```python
from build123d import *

# Parameters (mm, degrees)
F3_R = 5


# Not quite as in the source:
# - a fillet or chamfer that OpenCascade refuses, or shapes differently, is made with other operations: its cross-section is extruded or revolved along the edge and cut away or added


with BuildPart() as f1:
    # F0 (on Front) → F1 (revolve)
    with BuildSketch(Plane.XZ):
        Polygon((4, 11.2420413941), (2, 11.2420413941), (1.5147400554, 6.2420413941), (2, 1.2420413941), (4, 1.2420413941), (2.3485091515, 6.2420413941), align=None)
    revolve(axis=Axis((0, 0, 6.2420413941), (0, 0, 1)))

    # F2: fillet of radius 1.5 on 2 edges, made by hand

    # F2_s1 → F2_t2 (revolve, cut)
    with BuildSketch(Plane.XZ):
        with BuildLine():
            ThreePointArc((3.3497763701, 9.2734454721), (3.162587688, 10.592136722), (2, 11.2420413941))
            Line((2, 11.2420413941), (4, 11.2420413941))
            Line((4, 11.2420413941), (3.3497763701, 9.2734454721))
        make_face()
    revolve(axis=Axis((0, 0, 11.2420413941), (0, 0, 1)), mode=Mode.SUBTRACT)

    # F2_s3 → F2_t4 (revolve, cut)
    with BuildSketch(Plane.XZ):
        with BuildLine():
            ThreePointArc((2, 1.2420413941), (3.162587688, 1.8919460662), (3.3497763701, 3.2106373161))
            Line((3.3497763701, 3.2106373161), (4, 1.2420413941))
            Line((4, 1.2420413941), (2, 1.2420413941))
        make_face()
    revolve(axis=Axis((0, 0, 1.2420413941), (0, 0, 1)), mode=Mode.SUBTRACT)

    # F3
    f3_edges = [f1.edges().sort_by_distance(p)[0] for p in [
        (-2.348509, 0, 6.242041),
    ]]
    fillet(f3_edges, radius=F3_R)


solid = f1.part
```
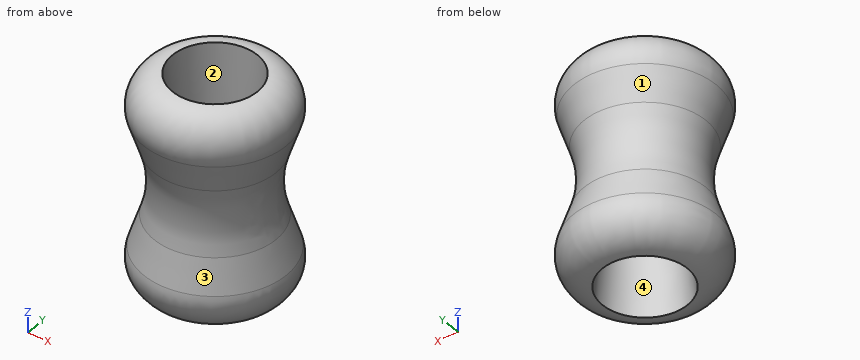
Geometry check sheet. Reference: the model listing, model coordinates, mm. Face numbers are marked on the shaded views. A direction names the side the tool comes from. Coordinates: 2 decimals unless noted, no trailing zeros. Order: outer loops, then holes, each group sorted by start corner. A loop starts at its lowest first (then second) coordinate and runs counter-clockwise, first axis right, second up. Notation, with made-up numbers: M -23,88 L 16,88 A28 ccw 16,106 Z; hole C -28,-28.75 d10. An arc over 180 degrees is marked long. Answer as a JSON object with one key per item and string values.
Q1. Cross-section at A-A on z = 8.25. Record the cut outline in (x, y), and give its area (3 significant figures).
Results are:
{"outline": "C 0,0 d6.02; hole C 0,0 d3.42", "area": "19.3 mm²"}
Q2. Tool access check on the marked faces 1 and 2. Record the directions out of +Z, -Z, +X, -X, +Y, -Y that give a thin tool (end or side, any length) a straight path to the whole face; none if there is none.
Results are:
{"face 1": "none", "face 2": "+Z"}
Q3. Cross-section at B-B on z = 3.75. Record the cut outline in (x, y).
Results are:
{"outline": "C 0,0 d6.34; hole C 0,0 d3.51"}
Q4. Scan lines: line 1 (X direction, y = -0.5, z = 2.25); line 2 (Y direction, x = -0.75, z = 5.25); line 3 (Y direction, x = -1.25, z = 8.75). Record each from-to range of solid material in increasing order.
Results are:
{"line 1": "x = -3.31 to -1.84, 1.84 to 3.31", "line 2": "y = -2.61 to -1.43, 1.43 to 2.61", "line 3": "y = -2.92 to -1.24, 1.24 to 2.92"}
Q5. Depth check by flat-ended pin: pin 1 Ø3 at (y, z) = (-1.5, 7) entering from -X; pin 2 Ø2 at (x, z) = (-2.5, 7) entering from -Y; pin 3 Ø1.5 at (y, z) = (0.5, 8) entering from +X. Enter the tip coordinate at first touch or a pass-through.
Results are:
{"pin 1": "stops at x = -2.94", "pin 2": "stops at y = -2.25", "pin 3": "stops at x = 3.15"}
Q6. Release check for a two-part mould opening along X. For the marked faces 3 and 4 record: released by +X, released by -X, zero draft, split by the parting line, or undercut.
Results are:
{"face 3": "split by the parting line", "face 4": "undercut"}
